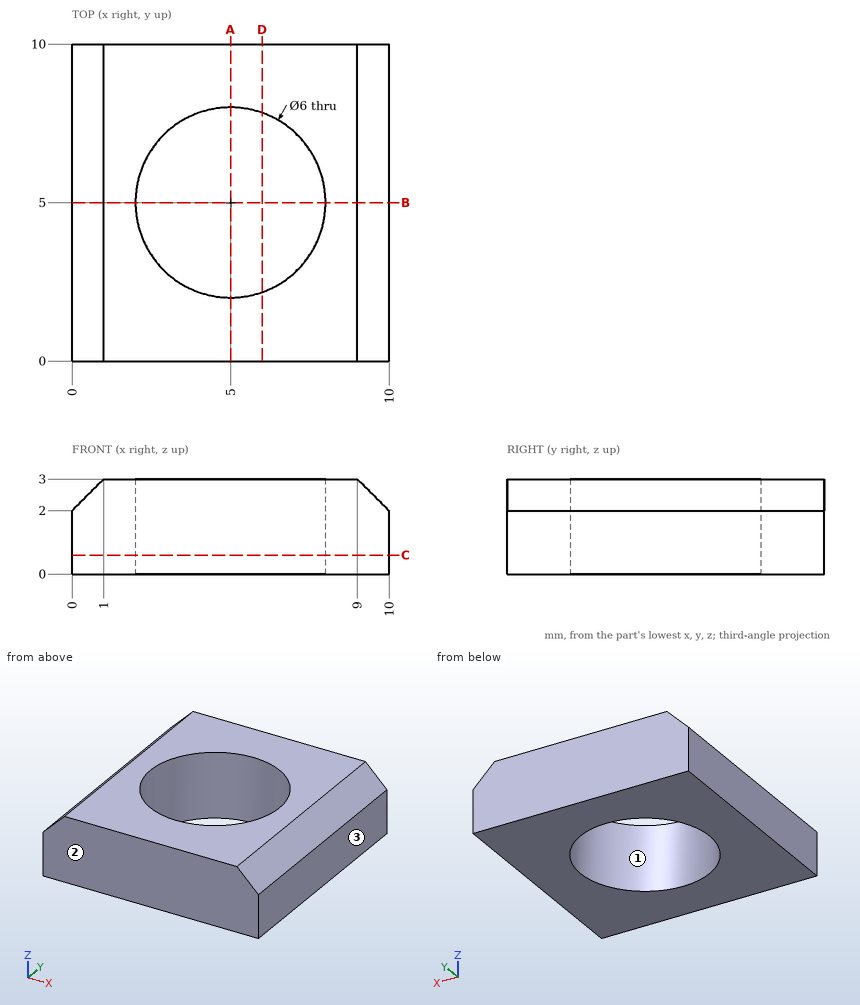
The figure shows three views and two pictorial views of one solid part (mm, origin at its lowest corner). Answer the questions. Give positions to 0.01 mm unless a question says otherwise; leave off trailing zeros. Loops run counter-clockwise (first coordinate to the right, second up) from the corner with the lowest first, then second, coordinate; pieces in that order, holes last. Notation, with made-up numbers: (-32, -17) -> (26, -17) arc R20 cw to (26, 11) -> close; hole circle Ø8 at (-27, 31). An arc over 180 degrees is marked (long way). Use a Markdown table: item, result. Add a question column.
1. Section A-A on x = 5 is taken. Determine the outline of the cut face in (y, z), and give its area (3 significant figures).
2. Find the intervals of material crossed by probe 1 along Y at (x, z) = (5, 1.9); probe 2 along X at (y, z) = (5.75, 2.55); probe 3 along X at (y, z) = (2.75, 1.85), in increasing order.
3. Determine the mould class of the marked faces 1, 2 and 3 for opening direction X: released by +X, released by -X, zero draft, split by the parting line, or undercut.
4. Section D-D on x = 6 is taken. Determine the outline of the cut face in (y, z), and give its area (3 significant figures).
5. Section C-C on z = 0.6 is taken. Determine the outline of the cut face in (x, y), and give its area (3 significant figures).
6. A flat-ended cylindrical pin translates along its axis: pin 1 Ø5.5 at (x, y) = (5, 5) entering from +Z. Find the tip coordinate at first contact, or state that the pin passes through.
7. Section B-B on y = 5 is taken. Determine the outline of the cut face in (x, z), and give its area (3 significant figures).
Results below:
| question | item | result |
|---|---|---|
| 1 | outline | (0, 0) -> (2, 0) -> (2, 3) -> (0, 3) -> close; (8, 0) -> (10, 0) -> (10, 3) -> (8, 3) -> close |
| 1 | area | 12.0 mm^2 |
| 2 | probe 1 | y = 0 to 2, 8 to 10 |
| 2 | probe 2 | x = 0.55 to 2.1, 7.9 to 9.45 |
| 2 | probe 3 | x = 0 to 3.02, 6.98 to 10 |
| 3 | face 1 | undercut |
| 3 | face 2 | zero draft |
| 3 | face 3 | released by +X |
| 4 | outline | (0, 0) -> (2.17, 0) -> (2.17, 3) -> (0, 3) -> close; (7.83, 0) -> (10, 0) -> (10, 3) -> (7.83, 3) -> close |
| 4 | area | 13.0 mm^2 |
| 5 | outline | (0, 0) -> (10, 0) -> (10, 10) -> (0, 10) -> close; hole circle Ø6 at (5, 5) |
| 5 | area | 71.7 mm^2 |
| 6 | pin 1 | passes through |
| 7 | outline | (0, 0) -> (2, 0) -> (2, 3) -> (1, 3) -> (0, 2) -> close; (8, 0) -> (10, 0) -> (10, 2) -> (9, 3) -> (8, 3) -> close |
| 7 | area | 11.0 mm^2 |
